CAD build for the part. Positions are in the model's coordinates, mm. A direction names the side the tool comes from. Round coordinates to 2 decimals unless told otherwise and drop trailing zeros. Use one line per item in the form item = value. Start each with the question number.
Item 1: Tool access for faces 1 (the cylindrical face through (248.9, -82.9, 95.1)), 2 (the flat face through (-249, -82, 105)), 3 (the flat face through (147.49, -75.81, 56.42)), 4 (the flat face through (230, -77, 80)), 5 (the flat face through (-53, -27, 23.15)): list every direction of +Z, -Z, +X, -X, +Y, -Y with a clear straight run to the whole face (end or side of a thin tool).
Item 2: Drill centre lines: L1, parallel to Y at x = 50, z = 25; L2, parallel to X at y = -97, z = 100; L3, parallel to X at y = -88, z = 101.5. Where is each one in solid material? Low to high.
Item 3: Pin check, flat tips, straight feed: pin 1 (15.5 mm diameter, centred on x = -20, z = 10.5, fed in from +Y); pin 2 (6 mm diameter, centred on x = 17.5, z = 35, fed in from +Y); pin 3 (6 mm diameter, centred on y = -57, z = 60.5, fed in from -X); pin 4 (0.8 mm diameter, centred on y = -149, z = 96.5, fed in from -X). Stop position of each tip, or through.
Item 4: Pull direction X, two halves, no side cores. Call faces 6 (the cylindrical face through (187.891, -98.929, 78.074)), 7 (the flat face through (227, -79, 110)), 8 (the cylindrical face through (239.76, -146.31, 84.79)): +X half, -X half, draft (parallel to the pull), parting line (faces both ways), or undercut.
from build123d import *

# Parameters (mm, degrees)
EXTRUDE_THIN1_DEPTH                       = 150
SKETCH2_OUTSIDE_W                         = 349.23
SKETCH2_OUTSIDE_H                         = 219.23
CUT_EXTRUDE1_DEPTH                        = 337.154726279
SKETCH3_R                                 = 30
CUT_EXTRUDE2_DEPTH                        = 323.116973634
CUT_EXTRUDE3_START                        = -15
CUT_EXTRUDE3_DEPTH                        = 10
SKETCH5_W                                 = 100
SKETCH5_H                                 = 2
CUT_EXTRUDE4_DEPTH                        = 323.116973634
CBORE_START                               = 14.1
CBORE_SLOT_FOR_M24_HEX_HEAD_BOLT1_DEPTH   = 15.9
CBORE_SLOT_FOR_M24_HEX_HEAD_BOLT1_2_DEPTH = 14.1
CBORE_FOR_M10_HEX_HEAD_BOLT1_D            = 11
CBORE_FOR_M10_HEX_HEAD_BOLT1_CBORE_D      = 21.48
CBORE_FOR_M10_HEX_HEAD_BOLT1_CBORE_DEPTH  = 6.85
CUT_EXTRUDE5_DEPTH                        = 303.31664336
FILLET1_R                                 = 40


# Read off the part's stored shape, not the designer's step: CBORE SLOT for M24 Hex Head Bolt1
with BuildPart() as part:
    # Sketch1 → Extrude-Thin1 (new body)
    with BuildSketch(Plane(origin=(0, 0, 0), x_dir=(1, 0, 0), z_dir=(0, 1, 0))):
        with BuildLine():
            Line((0, 0), (-96.684617092, 0))
            ThreePointArc((-96.684617092, 0), (-117.815530179, -4.684610648), (-134.986839248, -17.860619516))
            Line((-134.986839248, -17.860619516), (-181.133234795, -72.855752194))
            ThreePointArc((-181.133234795, -72.855752194), (-188.001758422, -78.126155741), (-196.454123657, -80))
            Line((-196.454123657, -80), (-280, -80))
            Line((-280, -80), (-280, -110))
            Line((-280, -110), (-196.454123657, -110))
            ThreePointArc((-196.454123657, -110), (-175.32321057, -105.315389352), (-158.151901501, -92.139380484))
            Line((-158.151901501, -92.139380484), (-112.005505955, -37.144247806))
            ThreePointArc((-112.005505955, -37.144247806), (-105.136982327, -31.873844259), (-96.684617092, -30))
            Line((-96.684617092, -30), (0, -30))
            Line((0, -30), (0, 0))
        make_face()
    extrude(amount=-EXTRUDE_THIN1_DEPTH)

    # Sketch2 outside → Cut-Extrude1 (cut, through all)
    with BuildSketch(Plane.XY):
        with Locations((-140, -75)):
            Rectangle(SKETCH2_OUTSIDE_W, SKETCH2_OUTSIDE_H)
        with BuildLine():
            Line((0, 0), (-234.676511429, -71.747809761))
            ThreePointArc((-234.676511429, -71.747809761), (-261.233833478, -121.694868189), (-211.286775051, -148.252190239))
            Line((-211.286775051, -148.252190239), (-95, -112.699755258))
            add(Edge.make_bspline(
                [(-95, -112.699755258), (-51.532544729, -99.410420536), (-36.95554526, -100), (0, -100)],
                knots=[0, 0, 0, 0, 1, 1, 1, 1], degree=3))
            Line((0, -100), (0, 0))
        make_face(mode=Mode.SUBTRACT)
    extrude(amount=CUT_EXTRUDE1_DEPTH, mode=Mode.SUBTRACT)

    # Sketch3 → Cut-Extrude2 (cut, through all)
    with BuildSketch(Plane.XY.offset(110)):
        with Locations(Location((-222.98164324, -110, 0), (0, 0, 27.840553026))):
            Circle(SKETCH3_R)
    extrude(amount=-CUT_EXTRUDE2_DEPTH, mode=Mode.SUBTRACT)

    # Sketch4 → Cut-Extrude3 (cut, symmetric)
    with BuildSketch(Plane.XY.offset(110).offset(CUT_EXTRUDE3_START)):
        with BuildLine():
            Line((-222.98164324, -68.172329741), (-222.98164324, -72.5))
            ThreePointArc((-222.98164324, -72.5), (-260.48164324, -110), (-222.98164324, -147.5))
            Line((-222.98164324, -147.5), (-222.98164324, -150))
            ThreePointArc((-222.98164324, -150), (-262.542277774, -115.912376445), (-234.676511429, -71.747809761))
            Line((-234.676511429, -71.747809761), (-222.98164324, -68.172329741))
        make_face()
    extrude(amount=CUT_EXTRUDE3_DEPTH, both=True, mode=Mode.SUBTRACT)

    # Sketch5 → Cut-Extrude4 (cut, through all)
    with BuildSketch(Plane.XY.offset(110)):
        with Locations((-272.98164324, -110)):
            Rectangle(SKETCH5_W, SKETCH5_H)
    extrude(amount=-CUT_EXTRUDE4_DEPTH, mode=Mode.SUBTRACT)

    # CBORE SLOT for M24 Hex Head Bolt1 outlin → CBORE SLOT for M24 Hex Head Bolt1 (cut)
    with BuildSketch(Plane.XY.offset(CBORE_START)):
        with BuildLine():
            Line((0, -47.715), (-47, -47.715))
            ThreePointArc((-47, -47.715), (-69.285, -70), (-47, -92.285))
            Line((-47, -92.285), (0, -92.285))
            Line((0, -92.285), (0, -47.715))
        make_face()
    extrude(amount=CBORE_SLOT_FOR_M24_HEX_HEAD_BOLT1_DEPTH, mode=Mode.SUBTRACT)

    # CBORE SLOT for M24 Hex Head Bolt1 2 outl → CBORE SLOT for M24 Hex Head Bolt1 2 (cut)
    with BuildSketch(Plane.XY):
        with BuildLine():
            Line((0, -83), (0, -57))
            Line((0, -57), (-47, -57))
            ThreePointArc((-47, -57), (-60, -70), (-47, -83))
            Line((-47, -83), (0, -83))
        make_face()
    extrude(amount=CBORE_SLOT_FOR_M24_HEX_HEAD_BOLT1_2_DEPTH, mode=Mode.SUBTRACT)

    # CBORE for M10 Hex Head Bolt1 (through all)
    with Locations(Plane.XY.offset(30)):
        with Locations((-50, -32)):
            CounterBoreHole(CBORE_FOR_M10_HEX_HEAD_BOLT1_D / 2, CBORE_FOR_M10_HEX_HEAD_BOLT1_CBORE_D / 2, CBORE_FOR_M10_HEX_HEAD_BOLT1_CBORE_DEPTH)

    # Sketch11 → Cut-Extrude5 (cut, through all)
    with BuildSketch(Plane(origin=(-47.437557366, 0, -39.80483689), x_dir=(0.6427876096865384, 0, -0.7660444431189788), z_dir=(0.7660444431189788, 0, 0.6427876096865384))):
        with BuildLine():
            Line((-159.78881321, -80.089014291), (-115.633379107, -71.411593064))
            ThreePointArc((-115.633379107, -71.411593064), (-106.827903218, -77.32459521), (-112.740905364, -86.130071099))
            Line((-112.740905364, -86.130071099), (-156.896339468, -94.807492326))
            ThreePointArc((-156.896339468, -94.807492326), (-165.701815356, -88.89449018), (-159.78881321, -80.089014291))
        make_face()
    extrude(amount=-CUT_EXTRUDE5_DEPTH, mode=Mode.SUBTRACT)

    # Mirror1: part across plane


with BuildPart() as part_1:
    add(part.part)
    add(part.part.mirror(Plane(origin=(0, -150, 0), x_dir=(0, 0, 1), z_dir=(-1, 0, 0))))

    # Fillet1
    fillet1_edges = [part_1.edges().sort_by_distance(p)[0] for p in [
        (0, 0, 15),
    ]]
    fillet(fillet1_edges, radius=FILLET1_R)


solid = part_1.part
Determined:
q1.face_1 = +X, +Y
q1.face_2 = -X, +Y
q1.face_3 = none
q1.face_4 = -Z, +X, +Y, -Y
q1.face_5 = +Z
q2.L1 = -101.98 to -92.08, -47.92 to -42.74, -21.26 to -15.29
q2.L2 = -258.16 to -250.02, -195.94 to -166.45, 166.45 to 195.94, 250.02 to 258.16
q2.L3 = -253.35 to -243.38, -202.59 to -168.57, 168.57 to 202.59, 243.38 to 253.35
q3.pin_1 = -3.75
q3.pin_2 = through
q3.pin_3 = -173.28
q3.pin_4 = -222.98
q4.face_6 = +X half
q4.face_7 = draft
q4.face_8 = undercut
